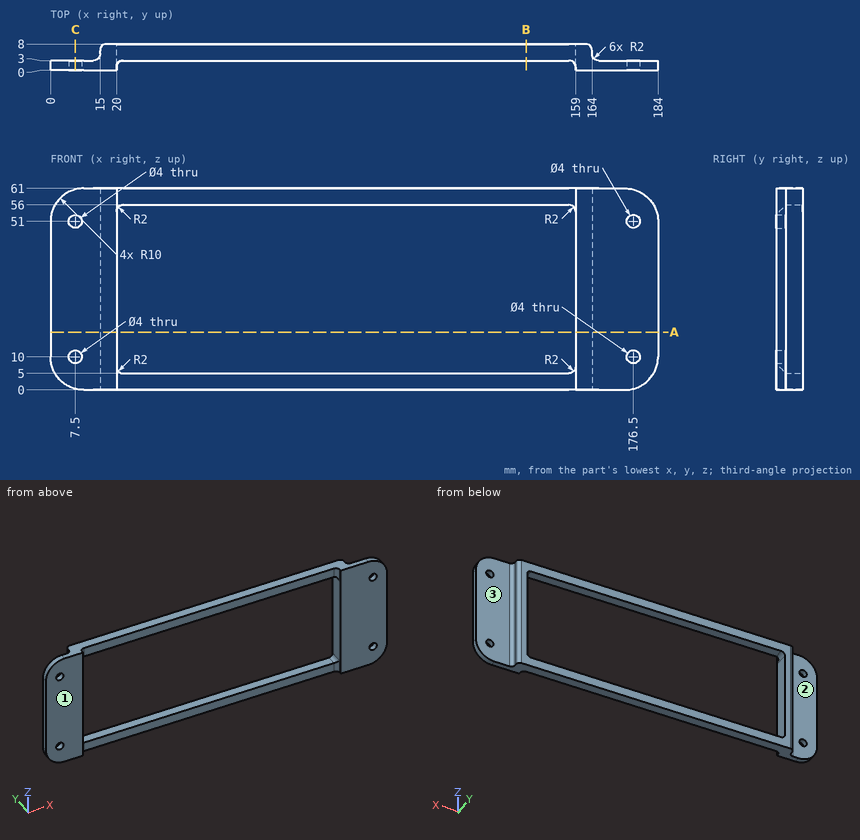
The drawing under review shows one solid part. Ordinate dimensions are in mm from its lowest x, y, z. A direction names the side the tool comes from. Coordinates: 2 decimals unless noted, no trailing zeros. Write each loop counter-clockwise with the first axis right and the second up, starting at its lowest first coordinate (ties: lowest second). Pieces come first, ordered by that corner, then holes. Notation, with made-up numbers: (71, 86.25) -> (81, 86.25) arc R23 cw to (81, 116.25) -> close; hole circle Ø3 at (27.5, 57.25). An arc over 180 degrees is marked (long way). Write each question's results on one line, items separated by ' | '. Start each with the question number.
1) Insertion check: pin 1 (6.5 mm diameter, centred on x = 7.5, z = 51, fed in from +Y); pin 2 (0.5 mm diameter, centred on y = 5.5, z = 39, fed in from +X); pin 3 (3 mm diameter, centred on x = 176.5, z = 10, fed in from -Y); pin 4 (2.5 mm diameter, centred on x = 98.5, z = 58, fed in from -Y). Each pin has a flat end and moves straight along its axis. Give the tip position at first contact, or say it passes through.
2) For the marked faces 1, 2 and 3, list the 3-axis set-ups (+Z, -Z, +X, -X, +Y, -Y) from which the entire face can be reached by the end or side of a thin tool; tool diameter is ignored.
3) Consider section C-C (x = 7.5). Write out the cut boundary in (y, z).
4) Consider section A-A (z = 17.5). Write out the cut boundary in (x, y).
5) Wall thickness on L1, parallel to X at y = 1.2, z = 10; L2, parallel to Z at x = 41, y = 6; L3, parallel to X at y = 1.5, z = 44.5: over which ranges is each line inside the solid? List them lowest first. Write a range as [from, to].
6) Consider section B-B (x = 144). Write out the cut boundary in (y, z).
Geometry says:
1) pin 1: y = 3 | pin 2: x = 164 | pin 3: through | pin 4: y = 3
2) face 1: +Z, -Z, +X, -X, -Y | face 2: +Z, -Z, -X, +Y | face 3: +Z, -Z, +X, +Y
3) outline: (0, 0.32) -> (3, 0.32) -> (3, 8) -> (0, 8) -> close; (0, 12) -> (3, 12) -> (3, 49) -> (0, 49) -> close; (0, 53) -> (3, 53) -> (3, 60.68) -> (0, 60.68) -> close
4) outline: (0, 0) -> (20, 0) -> (20, 8) -> (17, 8) arc R2 ccw to (15, 6) -> (15, 5) arc R2 cw to (13, 3) -> (0, 3) -> close; (159, 0) -> (184, 0) -> (184, 3) -> (166, 3) arc R2 cw to (164, 5) -> (164, 6) arc R2 ccw to (162, 8) -> (159, 8) -> close
5) L1: [0, 5.5], [9.5, 20], [159, 174.5], [178.5, 184] | L2: [0, 5], [56, 61] | L3: [0, 20], [159, 184]
6) outline: (3, 0) -> (8, 0) -> (8, 5) -> (3, 5) -> close; (3, 56) -> (8, 56) -> (8, 61) -> (3, 61) -> close
